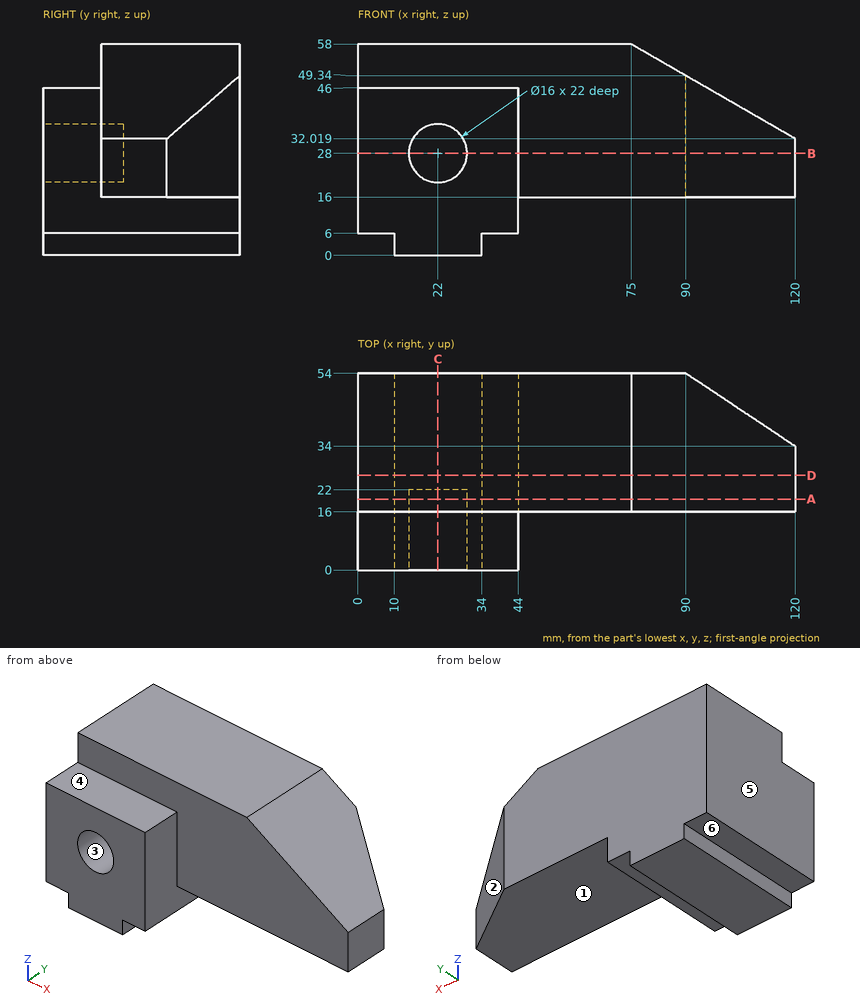
Here's the drawing with two shaded views (mm, measured from the low corner). I have some questions. A direction names the side the tool comes from. Give positions to 0.01 mm unless a question says otherwise; leave off trailing zeros. Loops run counter-clockwise (first coordinate to the right, second up) from the corner with the lowest first, then second, coordinate; pieces in that order, holes last. Notation, with made-up numbers: M 27.5,-39 L 80.5,-39 A14 cw 80.5,-12 Z; hole C -21.75,-14 d6. An arc over 180 degrees is marked long. One line per item, written item: value. Start each with the question number.
1) On a 3-axis mill with a long thin cutter (end or side, diameter ignored), from which of +Z, -Z, +X, -X, +Y, -Y can I reach the whole of each face in a straight line? I mean the marked faces 1 and 2. Say none if no direction works.
2) If we section it at C-C, the plane x = 22: Write out the boundary of the cut face in (y, z), and give its area (3 significant figures).
3) Thinking about a two-plate mould opening in Z: for the marked faces 3, 4, 5 and 6, which applies, +Z half, -Z half, draft (parallel to the pull), parting line (faces both ways), or undercut?
4) I'm going to push flat-ended pins straight in: pin 1 (6.5 mm diameter, centred on y = 22, z = 2.5, fed in from -X); pin 2 (8 mm diameter, centred on x = 19, z = 26, fed in from -Y); pin 3 (5 mm diameter, centred on y = 25.5, z = 4, fed in from +X). Where does each tip first touch, or does it pass through?
5) If we section it at D-D, the plane y = 26: Write out the boundary of the cut face in (x, z), and give its area (3 significant figures).
6) If we section it at B-B, the plane z = 28: Write out the boundary of the cut face in (x, y).
7) If we section it at A-A, the plane y = 19.5: Write out the boundary of the cut face in (x, z), and give its area (3 significant figures).
8) If I drill on line 1 (Z direction, x = 22, y = 9); line 2 (Z direction, x = 22, y = 16.5); line 3 (X direction, y = 2, z = 39.5), over which ranges is the centre line in solid material (lowest first)? Write a range as [from, to].
Completed:
1. face 1: -Z, +X, +Y, -Y
1. face 2: +Z, -Z, +X, +Y
2. outline: M 0,0 L 54,0 L 54,58 L 16,58 L 16,46 L 0,46 L 0,36 L 22,36 L 22,20 L 0,20 Z
2. area: 2,590 mm^2
3. face 3: undercut
3. face 4: +Z half
3. face 5: draft
3. face 6: -Z half
4. pin 1: stops at x = 10
4. pin 2: stops at y = 22
4. pin 3: stops at x = 44
5. outline: M 0,6 L 10,6 L 10,0 L 34,0 L 34,6 L 44,6 L 44,16 L 120,16 L 120,32.02 L 75,58 L 0,58 Z
5. area: 5,040 mm^2
6. outline: M 0,0 L 14,0 L 14,22 L 30,22 L 30,0 L 44,0 L 44,16 L 120,16 L 120,34 L 90,54 L 0,54 Z
7. outline: M 0,6 L 10,6 L 10,0 L 34,0 L 34,6 L 44,6 L 44,16 L 120,16 L 120,32.02 L 75,58 L 0,58 Z; hole C 22,28 d16
7. area: 4,840 mm^2
8. line 1: z = [0, 20], [36, 46]
8. line 2: z = [0, 20], [36, 58]
8. line 3: x = [0, 44]
